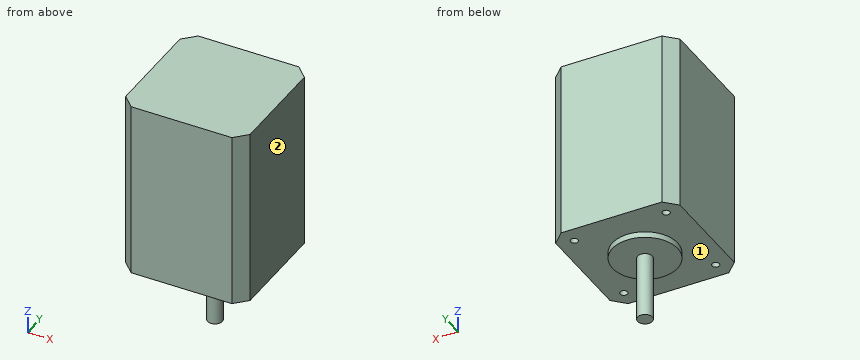
```python
from build123d import *

# Parameters (mm, degrees)
SKETCH_1_W               = 42
SKETCH_1_H               = 42
EXTRUDE_1_DEPTH          = 60
SKETCH_8_R               = 2.5
EXTRUDE_2_DEPTH          = 24
CUT_EXTRUDE_1_DEPTH      = 85
PATTERN_CIRCULAR_1_COUNT = 4
SKETCH_12_R              = 11
EXTRUDE_3_DEPTH          = 2


with BuildPart() as part:
    # Эскиз1 → Бобышка-Вытянуть1 (new body)
    with BuildSketch(Plane.XY):
        Rectangle(SKETCH_1_W, SKETCH_1_H)
    extrude(amount=EXTRUDE_1_DEPTH)

    # Эскиз8 → Бобышка-Вытянуть2 (add)
    with BuildSketch(Plane(origin=(0, 0, 0), x_dir=(-1, 0, 0), z_dir=(0, 0, -1))):
        Circle(SKETCH_8_R)
    extrude(amount=EXTRUDE_2_DEPTH)

    # Эскиз9 → Отверстие обработанное метчиком M32 (revolve, cut)
    with BuildSketch(Plane(origin=(-15.5, -15.5, 0), x_dir=(0, 1, 0), z_dir=(1, 0, 0))):
        Polygon((0, 0), (0, 8.251075774), (1.25, 7.5), (1.25, 0), align=None)
    hole_wizard_m32 = revolve(axis=Axis((-15.5, -15.5, -6.35), (0, 0, 1)), mode=Mode.SUBTRACT)

    # Эскиз3 → Вырез-Вытянуть1 (cut, through all)
    with BuildSketch(Plane.XY.offset(60)):
        Polygon((-21, 17), (-17, 21), (-21, 21), align=None)
    cut_extrude_1 = extrude(amount=-CUT_EXTRUDE_1_DEPTH, mode=Mode.SUBTRACT)

    # Круговой массив1: Отверстие обработанное метчиком M32, Вырез-Вытянуть1 ×4 about axis
    pattern_circular_1_axis = Axis((0, 0, 0), (0, 0, 1))
    for i in range(1, PATTERN_CIRCULAR_1_COUNT):
        add(hole_wizard_m32.rotate(pattern_circular_1_axis, i * 360 / PATTERN_CIRCULAR_1_COUNT), mode=Mode.SUBTRACT)
        add(cut_extrude_1.rotate(pattern_circular_1_axis, i * 360 / PATTERN_CIRCULAR_1_COUNT), mode=Mode.SUBTRACT)

    # Эскиз12 → Бобышка-Вытянуть3 (add)
    with BuildSketch(Plane(origin=(0, 0, 0), x_dir=(-1, 0, 0), z_dir=(0, 0, -1))):
        Circle(SKETCH_12_R)
    extrude(amount=EXTRUDE_3_DEPTH)


solid = part.part
```
Could you check a few things on this model? Use its own coordinates, in mm. Face numbers are marked on the shaded views. A direction names the side the tool comes from. Round coordinates to 2 decimals unless told otherwise and drop trailing zeros. Loops run counter-clockwise (first coordinate to the right, second up) from the corner with the lowest first, then second, coordinate; pieces in that order, holes last. Notation, with made-up numbers: M -38,67 L 14,67 A27 cw 14,92 Z; hole C 62,21.5 d10. An arc over 180 degrees is marked long. Write item = value, one per line.
1. I want a section at D-D, the plane z = 13. Write out the boundary of the cut face in (x, y).
Results below:
outline = M -21,-17 L -17,-21 L 17,-21 L 21,-17 L 21,17 L 17,21 L -17,21 L -21,17 Z
2. I need wall thicknesses on probe 1 along Y at (x, z) = (-15.5, 2.75); probe 2 along Y at (x, z) = (15, 3). Which ranges of each line are inside material? Lowest first, please.
Results below:
probe_1 = -21 to -16.75, -14.25 to 14.25, 16.75 to 21
probe_2 = -21 to -16.65, -14.35 to 14.35, 16.65 to 21
3. I want a section at B-B, the plane x = 0. Write out the boundary of the cut face in (y, z), and give its area (3 significant figures).
Results below:
outline = M -21,0 L -11,0 L -11,-2 L -2.5,-2 L -2.5,-24 L 2.5,-24 L 2.5,-2 L 11,-2 L 11,0 L 21,0 L 21,60 L -21,60 Z
area = 2,670 mm²
4. Which directions (+Z, -Z, +X, -X, +Y, -Y) give clear straight access to the entire face, cutting with the end or side of a thin tool? Please do the marked faces 1 and 2.
Results below:
face_1 = -Z
face_2 = +Z, -Z, +X, +Y, -Y
5. I want a section at A-A, the plane z = 3.5. Write out the boundary of the cut face in (x, y), and give its area (3 significant figures).
Results below:
outline = M -21,-17 L -17,-21 L 17,-21 L 21,-17 L 21,17 L 17,21 L -17,21 L -21,17 Z; hole C -15.5,-15.5 d2.5; hole C -15.5,15.5 d2.5; hole C 15.5,-15.5 d2.5; hole C 15.5,15.5 d2.5
area = 1,710 mm²
6. Will these pins go through, and if not, where does the flat tip stop? P1, Ø6.5, axis at x = 0.5, y = -3.5, coming from the -Z side; P2, Ø4, axis at x = 14, y = -11, coming from the -Z side; P3, Ø2, axis at x = 15.5, y = 15.5, coming from the -Z side; P4, Ø10, axis at y = -15.5, z = -8, coming from the +X side.
Results below:
P1 = -24
P2 = 0
P3 = 7.65
P4 = through
